Geometry: final body of the model. Coordinates: model frame, mm. A direction names the side the tool comes from. Give positions to 0.01 mm unless a question says otherwise; leave off trailing zeros.
Q1. Pin query (flat end, axial travel): pin 1 Ø1 at (y, z) = (-2, -1) entering from +X; pin 2 Ø1 at (y, z) = (-1.5, -2) entering from -X. Return the tip coordinate at first contact, or that it passes through.
Q2. Line query: line 1 (Z direction, x = 1, y = -12.25); line 2 (Y direction, x = 2, z = 0.5); line 3 (X direction, y = -7, z = 2.5). Output: solid intervals per line, ascending.
Q3. Reachability of faces 1 (the cylindrical face through (-0.54, -2.71, -2.44)), 2 (the flat face through (1, 0, 0)) from +Z, -Z, +X, -X, +Y, -Y: full face, straight path, thin tool, end or side. Return the list, or none.
from build123d import *

# Parameters (mm, degrees)
F0_R     = 2.5
F1_DEPTH = 5.5
F2_R     = 2.5
F3_DEPTH = 3.5
F7_DEPTH = 25


# Not quite as in the source:
# - the arcs of a loft's sections are written as splines that run evenly, so that the points pair up as in the source's solid


with BuildPart() as f1:
    # F0 (on Front) → F1 (new body)
    with BuildSketch(Plane.XZ):
        Circle(F0_R)
    extrude(amount=F1_DEPTH)

    # F2 (on face) → F3 (join)
    with BuildSketch(Plane.XZ.offset(5.5)):
        Polygon((3, -1.7320508076), (3, 1.7320508076), (0, 3.4641016151), (-3, 1.7320508076), (-3, -1.7320508076), (0, -3.4641016151), align=None)
        Circle(F2_R, mode=Mode.SUBTRACT)
        Circle(F2_R)
    extrude(amount=F3_DEPTH)

    # F5 (on offset) → F6 section 0
    with BuildSketch(Plane.XZ.offset(14)):
        with BuildLine():
            add(Edge.make_bspline(
                [(0.1732050808, -0.1), (0.1848406091, -0.0798466737), (0.192920574, -0.0576471526), (0.2010025272, -0.0118121185), (0.2010025272, 0.0118121185), (0.192920574, 0.0576471526), (0.1848406091, 0.0798466737), (0.1732050808, 0.1)],
                knots=[0, 0, 0, 0, 0.3333333333, 0.3333333333, 0.6666666667, 0.6666666667, 1, 1, 1, 1], degree=3))
            add(Edge.make_bspline(
                [(0.1732050808, 0.1), (0.1615695524, 0.1201533263), (0.1463841856, 0.1382505417), (0.1107308583, 0.1681672355), (0.0902716689, 0.179979354), (0.0465363884, 0.1958976943), (0.0232710567, 0.2), (0, 0.2)],
                knots=[0, 0, 0, 0, 0.3333333333, 0.3333333333, 0.6666666667, 0.6666666667, 1, 1, 1, 1], degree=3))
            add(Edge.make_bspline(
                [(0, 0.2), (-0.0232710567, 0.2), (-0.0465363884, 0.1958976943), (-0.0902716689, 0.179979354), (-0.1107308583, 0.1681672355), (-0.1463841856, 0.1382505417), (-0.1615695524, 0.1201533263), (-0.1732050808, 0.1)],
                knots=[0, 0, 0, 0, 0.3333333333, 0.3333333333, 0.6666666667, 0.6666666667, 1, 1, 1, 1], degree=3))
            add(Edge.make_bspline(
                [(-0.1732050808, 0.1), (-0.1848406091, 0.0798466737), (-0.192920574, 0.0576471526), (-0.2010025272, 0.0118121185), (-0.2010025272, -0.0118121185), (-0.192920574, -0.0576471526), (-0.1848406091, -0.0798466737), (-0.1732050808, -0.1)],
                knots=[0, 0, 0, 0, 0.3333333333, 0.3333333333, 0.6666666667, 0.6666666667, 1, 1, 1, 1], degree=3))
            add(Edge.make_bspline(
                [(-0.1732050808, -0.1), (-0.1615695524, -0.1201533263), (-0.1463841856, -0.1382505417), (-0.1107308583, -0.1681672355), (-0.0902716689, -0.179979354), (-0.0465363884, -0.1958976943), (-0.0232710567, -0.2), (0, -0.2)],
                knots=[0, 0, 0, 0, 0.3333333333, 0.3333333333, 0.6666666667, 0.6666666667, 1, 1, 1, 1], degree=3))
            add(Edge.make_bspline(
                [(0, -0.2), (0.0232710567, -0.2), (0.0465363884, -0.1958976943), (0.0902716689, -0.179979354), (0.1107308583, -0.1681672355), (0.1463841856, -0.1382505417), (0.1615695524, -0.1201533263), (0.1732050808, -0.1)],
                knots=[0, 0, 0, 0, 0.3333333333, 0.3333333333, 0.6666666667, 0.6666666667, 1, 1, 1, 1], degree=3))
        make_face()
    # F3_face (on face) → F6 section 1
    with BuildSketch(Plane.XZ.offset(9)):
        Polygon((3, -1.7320508076), (3, 1.7320508076), (0, 3.4641016151), (-3, 1.7320508076), (-3, -1.7320508076), (0, -3.4641016151), align=None)
    loft(ruled=True)

    # F7 (cut): a face of the model
    f7_faces = [f1.faces().sort_by_distance(p)[0] for p in [
        (0, -14, 0),
    ]]
    extrude(f7_faces, amount=-F7_DEPTH, mode=Mode.SUBTRACT)


solid = f1.part
Computed:
1. pin 1: stops at x = 2.45
1. pin 2: stops at x = -2
2. line 1: z = -0.77 to 0.77
2. line 2: y = -10.78 to 0
2. line 3: x = -1.67 to 1.67
3. face 1: +Y
3. face 2: +Z, -Z, +X, -X, +Y
